For this review, take the finished solid that the model builds, in its own axes (mm). A direction names the side the tool comes from. Round coordinates to 2 decimals unless told otherwise and drop trailing zeros. Write each loop counter-clockwise with the first axis right and the second up, starting at its lowest first coordinate (ties: lowest second). Pieces come first, ordered by that corner, then holes. Notation, with made-up numbers: (9.5, 62.5) -> (51.5, 62.5) arc R15 cw to (51.5, 80.5) -> close; hole circle Ø2 at (-4.5, 52). An arc over 180 degrees is marked (long way). Answer in a Markdown table with one row per item.
from build123d import *
from OCP.BRepFilletAPI import BRepFilletAPI_MakeChamfer

# Parameters (mm, degrees)
SKETCH1_R                = 1.6
SKETCH1_W                = 16
SKETCH1_H                = 16
BOSS_EXTRUDE1_DEPTH      = 8
SKETCH2_W                = 16
SKETCH2_H                = 4
CUT_EXTRUDE1_DEPTH       = 40
FILLET1_R                = 4
BOSS_EXTRUDE5_DEPTH      = 8
BOSS_EXTRUDE5_DEPTH_BACK = 1
SKETCH3_W                = 32
SKETCH3_H                = 5
CHAMFER1_SIZE            = 3
CHAMFER2_SIZE            = 8
CHAMFER2_SIZE2           = 10
SKETCH5_W                = 12
SKETCH5_H                = 5
BOSS_EXTRUDE7_DEPTH      = 8
FILLET2_R                = 4
SKETCH6_R                = 1.6
CUT_EXTRUDE2_DEPTH       = 20
SKETCH7_R                = 3.05
CUT_EXTRUDE3_DEPTH       = 9
SKETCH8_R                = 3.05
BOSS_EXTRUDE8_DEPTH      = 5
BOSS_EXTRUDE9_START      = -5
SKETCH9_R                = 1.6
BOSS_EXTRUDE9_DEPTH      = 5
SKETCH10_R               = 5.5
CUT_EXTRUDE4_DEPTH       = 9
CUT_EXTRUDE5_DEPTH       = 37


with BuildPart() as part:
    # Sketch1 → Boss-Extrude1 (new body)
    with BuildSketch(Plane(origin=(0, 0, 0), x_dir=(1, 0, 0), z_dir=(0, 1, 0))):
        with BuildLine():
            Line((-12, 16), (12, 16))
            ThreePointArc((12, 16), (14.828427125, 14.828427125), (16, 12))
            Line((16, 12), (16, -12))
            ThreePointArc((16, -12), (14.828427125, -14.828427125), (12, -16))
            Line((12, -16), (-12, -16))
            ThreePointArc((-12, -16), (-14.828427125, -14.828427125), (-16, -12))
            Line((-16, -12), (-16, 12))
            ThreePointArc((-16, 12), (-14.828427125, 14.828427125), (-12, 16))
        make_face()
        with Locations(Location((12, 12, 0), (0, 0, 270))):
            Circle(SKETCH1_R, mode=Mode.SUBTRACT)
        with Locations(Location((-12, 12, 0), (0, 0, 90))):
            Circle(SKETCH1_R, mode=Mode.SUBTRACT)
        with Locations(Location((12, -12, 0), (0, 0, 90))):
            Circle(SKETCH1_R, mode=Mode.SUBTRACT)
        with Locations(Location((-12, -12, 0), (0, 0, 270))):
            Circle(SKETCH1_R, mode=Mode.SUBTRACT)
        Rectangle(SKETCH1_W, SKETCH1_H, mode=Mode.SUBTRACT)
    extrude(amount=BOSS_EXTRUDE1_DEPTH)

    # Sketch2 → Cut-Extrude1 (cut)
    with BuildSketch(Plane(origin=(16, 0, 0), x_dir=(0, 0, -1), z_dir=(1, 0, 0))):
        with Locations((0, 2)):
            Rectangle(SKETCH2_W, SKETCH2_H)
    extrude(amount=-CUT_EXTRUDE1_DEPTH, mode=Mode.SUBTRACT)

    # Fillet1
    fillet1_edges = [part.edges().sort_by_distance(p)[0] for p in [
        (-16, 2, -8),
        (16, 2, -8),
        (-16, 2, 8),
        (16, 2, 8),
    ]]
    fillet(fillet1_edges, radius=FILLET1_R - 0.0001)  # a hair under: the kernel refuses the full size

    # Sketch3 → Boss-Extrude5 (add, two sides: drawn at the far end of the back side and taken through both)
    with BuildSketch(Plane(origin=(0, 8, 0), x_dir=(1, 0, 0), z_dir=(0, 1, 0)).offset(-BOSS_EXTRUDE5_DEPTH_BACK)):
        with Locations((0, 5.5)):
            Rectangle(SKETCH3_W, SKETCH3_H)
        with Locations((0, -5.5)):
            Rectangle(SKETCH3_W, SKETCH3_H)
    extrude(amount=BOSS_EXTRUDE5_DEPTH + BOSS_EXTRUDE5_DEPTH_BACK)

    # Chamfer1
    chamfer1_edges = [part.edges().sort_by_distance(p)[0] for p in [
        (8, 7, 5.5),
        (8, 7, -5.5),
        (-8, 7, -5.5),
        (-8, 7, 5.5),
    ]]
    chamfer(chamfer1_edges, length=CHAMFER1_SIZE - 0.0001)  # a hair under: the kernel refuses the full size

    # Chamfer2: one chamfer whose edges measure the first distance from different faces: ONE call of the kernel's chamfer builder (chamfer() names one face for all edges)
    chamfer2_edges_1 = [part.edges().sort_by_distance(p)[0] for p in [
        (16, 16, -5.5),
        (16, 16, 5.5),
    ]]
    chamfer2_side_1 = [part.faces().sort_by_distance(p)[0] for p in [
        (16, 0.288444102, -11.99995),
    ]]
    chamfer2_edges_2 = [part.edges().sort_by_distance(p)[0] for p in [
        (-16, 16, -5.5),
        (-16, 16, 5.5),
    ]]
    chamfer2_side_2 = [part.faces().sort_by_distance(p)[0] for p in [
        (-16, 0.288444102, 11.99995),
    ]]
    chamfer2 = BRepFilletAPI_MakeChamfer(part.part.solid().wrapped)
    for e in chamfer2_edges_1:
        chamfer2.Add(CHAMFER2_SIZE, CHAMFER2_SIZE2, e.wrapped, chamfer2_side_1[0].wrapped)  # the first distance lies on this face
    for e in chamfer2_edges_2:
        chamfer2.Add(CHAMFER2_SIZE, CHAMFER2_SIZE2, e.wrapped, chamfer2_side_2[0].wrapped)  # the first distance lies on this face
    add(Compound.cast(chamfer2.Shape()), mode=Mode.REPLACE)

    # Sketch5 → Boss-Extrude7 (add)
    with BuildSketch(Plane(origin=(0, 16, 0), x_dir=(1, 0, 0), z_dir=(0, 1, 0))):
        with Locations((0, 5.5)):
            Rectangle(SKETCH5_W, SKETCH5_H)
        with Locations((0, -5.5)):
            Rectangle(SKETCH5_W, SKETCH5_H)
    extrude(amount=BOSS_EXTRUDE7_DEPTH)

    # Fillet2
    fillet2_edges = [part.edges().sort_by_distance(p)[0] for p in [
        (-6, 24, -5.5),
        (6, 24, -5.5),
        (-6, 24, 5.5),
        (6, 24, 5.5),
    ]]
    fillet(fillet2_edges, radius=FILLET2_R)

    # Sketch6 → Cut-Extrude2 (cut)
    with BuildSketch(Plane.XY.offset(8)):
        with Locations((0, 20)):
            Circle(SKETCH6_R)
    extrude(amount=-CUT_EXTRUDE2_DEPTH, mode=Mode.SUBTRACT)

    # Sketch7 → Cut-Extrude3 (cut)
    with BuildSketch(Plane.XY.offset(8)):
        with Locations((0, 20)):
            Circle(SKETCH7_R)
    extrude(amount=-CUT_EXTRUDE3_DEPTH, mode=Mode.SUBTRACT)

    # Sketch8 → Boss-Extrude8 (add)
    with BuildSketch(Plane.XY.offset(8)):
        with BuildLine():
            Line((-9, 20), (-9, 11))
            Line((-9, 11), (0, 11))
            Line((0, 11), (9, 11))
            Line((9, 11), (9, 20))
            ThreePointArc((9, 20), (0, 29), (-9, 20))
        make_face()
        with Locations((0, 20)):
            Circle(SKETCH8_R, mode=Mode.SUBTRACT)
    extrude(amount=-BOSS_EXTRUDE8_DEPTH)

    # Sketch9 → Boss-Extrude9 (add)
    with BuildSketch(Plane(origin=(0, 0, -8), x_dir=(-1, 0, 0), z_dir=(0, 0, -1)).offset(BOSS_EXTRUDE9_START)):
        with BuildLine():
            Line((-9, 20), (-9, 11))
            Line((-9, 11), (9, 11))
            Line((9, 11), (9, 20))
            ThreePointArc((9, 20), (0, 29), (-9, 20))
        make_face()
        with Locations(Location((0, 20, 0), (0, 0, 180))):
            Circle(SKETCH9_R, mode=Mode.SUBTRACT)
    extrude(amount=BOSS_EXTRUDE9_DEPTH)

    # Sketch10 → Cut-Extrude4 (cut)
    with BuildSketch(Plane(origin=(0, 0, -8), x_dir=(-1, 0, 0), z_dir=(0, 0, -1))):
        with Locations((0, 20)):
            Circle(SKETCH10_R)
    extrude(amount=-CUT_EXTRUDE4_DEPTH, mode=Mode.SUBTRACT)

    # Sketch11 → Cut-Extrude5 (cut)
    with BuildSketch(Plane(origin=(0, 8, 0), x_dir=(1, 0, 0), z_dir=(0, 1, 0))):
        Polygon((0, 3.1), (23.961552098, 3.1), (23.961552098, -3.1), (0, -3.1), (-29.391122595, -3.1), (-29.391122595, 3.1), align=None)
    extrude(amount=CUT_EXTRUDE5_DEPTH, mode=Mode.SUBTRACT)


solid = part.part
1) Consider section A-A on x = 0. State the section outline as (y, z) points.
Solved:
| item | result |
|---|---|
| outline | (0, -16) -> (8, -16) -> (8, -8) -> (14.5, -8) -> (14.5, -3.1) -> (8, -3.1) -> (8, -3) -> (7, -3) -> (7, -8) -> (0, -8) -> close; (0, 8) -> (7, 8) -> (7, 3) -> (8, 3) -> (8, 3.1) -> (16.95, 3.1) -> (16.95, 8) -> (8, 8) -> (8, 16) -> (0, 16) -> close; (23.05, 3.1) -> (29, 3.1) -> (29, 8) -> (23.05, 8) -> close; (25.5, -8) -> (29, -8) -> (29, -3.1) -> (25.5, -3.1) -> close |
2) Consider section B-B on y = 2.75. State how many separate pieces and enclosed holes the cut face has, then the cut area to 3 significant figures.
Solved:
| item | result |
|---|---|
| separate pieces | 2 |
| enclosed holes | 4 |
| area | 452 mm² |
3) Mouldability with a two-part tool opening along X and no side actions: class faces 1 (the flat face through (9, 17, -6)), 2 (the flat face through (0, 16, 3.1)), 3 (the flat face through (-0.1, 7.4, 3)) as pulls with the +X half, pulls with the -X half, needs draft (parallel to the pull), parting line crosses it, or undercut.
Solved:
| item | result |
|---|---|
| face 1 | pulls with the +X half |
| face 2 | needs draft |
| face 3 | undercut |
4) For line 1 (X direction, y = 2.25, z = -12); line 2 (Y direction, x = 0, z = 4.5); line 3 (Y direction, x = 0, z = -6.65), list the stretches that pass through material, from the lowest coordinate up. Write a range as [from, to].
Solved:
| item | result |
|---|---|
| line 1 | [-16, -13.6], [-10.4, 10.4], [13.6, 16] |
| line 2 | [7, 16.95], [23.05, 29] |
| line 3 | [7, 14.5], [25.5, 29] |
5) Clearance check with flat-ended pins moving along their axes: pin 1 Ø2 at (x, z) = (-12, -7) entering from +Y; pin 2 Ø4 at (x, z) = (13.5, -2) entering from -Y; pin 3 Ø4 at (x, z) = (4, -13) entering from +Y. State where each tip first meets the part, or that it passes through.
Solved:
| item | result |
|---|---|
| pin 1 | y = 12 |
| pin 2 | y = 4 |
| pin 3 | y = 8 |
6) Consider section C-C on z = -1. State the section outline as (x, y) points.
Solved:
| item | result |
|---|---|
| outline | (-16, 4) -> (-8, 4) -> (-8, 8) -> (-16, 8) -> close; (8, 4) -> (16, 4) -> (16, 8) -> (8, 8) -> close |
7) For faces 4 (the flat face through (-9, 17, -6)), 5 (the flat face through (-7, 5, 6)), 6 (the flat face through (11, 8, 0)), 7 (the flat face through (0, 16, 8)), list the 3-axis set-ups (+Z, -Z, +X, -X, +Y, -Y) from which the entire face can be reached by the end or side of a thin tool; tool diameter is ignored.
Solved:
| item | result |
|---|---|
| face 4 | +Z, -Z, -X, +Y |
| face 5 | -Y |
| face 6 | +X, -X, +Y |
| face 7 | +Z, +X, -X, +Y |
